Work out the finished part from the listing and answer in its coordinate system (mm). Face numbers are marked on the shaded views. A direction names the side the tool comes from. Coordinates: 2 decimals unless noted, no trailing zeros. Loops run counter-clockwise (first coordinate to the right, second up) from the corner with the lowest first, then second, coordinate; pieces in that order, holes last.
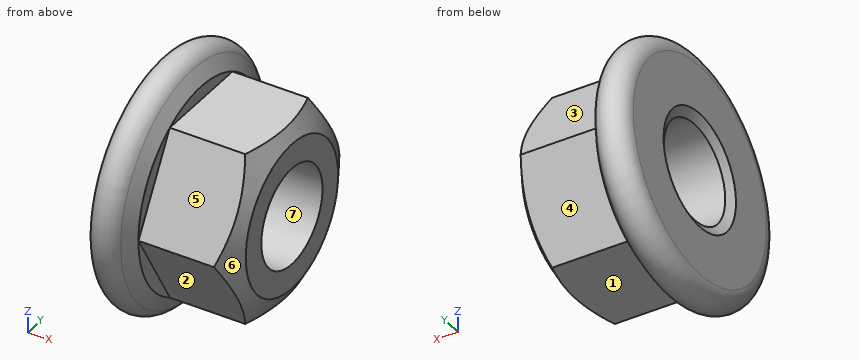
Autodesk Inventor part; units mm, degrees
ref_plane "Work Plane1" through (45.1755, 0, 0) normal (0, 0, -1) x (-1, 0, 0)
ref_plane "YZ Plane" through (0, 0, 0) normal (1, 0, 0) x (0, 1, 0)
ref_plane "XZ Plane" through (0, 0, 0) normal (0, 1, 0) x (-1, 0, 0)
sketch "Esquisse1" plane through (0, 0, 0) normal (0, 0, 1) x (1, 0, 0)
  line L0 (-3.6634, 0) -> (19.1606, 0)
  line L1 (4.9438, 12.1244) -> (3.9187, 13.9)
  line L2 (4.9438, 12.1244) -> (15.9, 12.1244) construction
  line L3 (15.9, 12.1244) -> (15.9, 0) construction
  arc A0 (3.9187, 13.9) -> (0, 12.85) centre (2.1, 12.85) ccw
  line L4 (4.9438, 12.1244) -> (4.9438, 0)
  line L5 (0, -3.0807) -> (0, 18.4841)
  point P0 (0, 0)
  dimension "d2" = 24.2487
  dimension "d4" = 29.9
  dimension "d5" = 2.1
  dimension "d15" = 15.9
  dimension "d16" = 30
revolve "Anneau" add sketch "Esquisse1" angle 360 about axis through (-10, 0, 0) along (1, 0, 0)
sketch "Esquisse2" plane through (0, 0, 0) normal (-1, 0, 0) x (0, 0, 1)
  circle A0 centre (0, 0) radius 4.9
  line L0 (-10.5, -6.0622) -> (-10.5, 6.0622)
  line L1 (-10.5, 6.0622) -> (0, 12.1244)
  line L2 (0, 12.1244) -> (10.5, 6.0622)
  line L3 (10.5, 6.0622) -> (10.5, -6.0622)
  line L4 (10.5, -6.0622) -> (0, -12.1244)
  line L5 (0, -12.1244) -> (-10.5, -6.0622)
  circle A1 centre (0, 0) radius 12.85
  dimension "d6" = 24.2487
extrude "Corps" add sketch "Esquisse2" against normal blind 15.9 contours A0 | L0 L1 L2 L3 L4 L5
sketch "Esquisse3" plane through (0, 0, 0) normal (0, 0, 1) x (1, 0, 0)
  line L0 (4.9438, 12.1244) -> (15.9, 12.1244)
  line L1 (15.9, 6.0622) -> (15.9, 12.1244)
  line L2 (0, -12.85) -> (0, 12.85)
  line L3 (-3.18, 0) -> (19.08, 0)
  line L4 (14.0529, 12.1244) -> (15.9, 8.925)
  dimension "d10" = 30
  dimension "d11" = 17.85
revolve "Chanfrein1" cut sketch "Esquisse3" angle 360 about axis through (-10, 0, 0) along (1, 0, 0)
sketch "Esquisse4" plane through (0, 0, 0) normal (-1, 0, 0) x (0, 0, 1)
  line L0 (-20.93, 0) -> (20.93, 0)
  line L1 (0, 20.93) -> (0, -20.93)
  point P0 (0, 0)
hole "Filetage" at (0, 0, 0) direction (1, 0, 0) diameter 11.835 end through all
chamfer "Chanfrein2" distance 1.0825 angle 30 1 edges at (0, 0, -5.9175) measured on face at (0, 10.4003, -1.2628)
ref_plane "Work Plane1" through (45.1755, 0, 0) normal (0, 0, -1) x (-1, 0, 0)
equation "\"d2\" = 1.1547 * SW"
equation "\"d4\" = LADI"
equation "\"d5\" = PHH"
equation "\"d15\" = KOH"
equation "\"d16\" = KEWI"
equation "\"d6\" = 1.1547 * SW"
equation "\"d7\" = KOH"
equation "\"d10\" = ANG1"
equation "\"d11\" = SW0"
equation "\"d12\" = -0.5 * GD1 + 0.5 * NND"
equation "\"d42\" = -0.5 * GD1 + 0.5 * NND"
equation "\"ANG1\" = 30deg"
equation "\"KEWI\" = 30deg"
equation "\"NND\" = 14"
equation "\"LADI\" = 29.9"
equation "\"SW\" = 21"
equation "\"PHH\" = 2.1"
equation "\"KOH\" = 15.9"
equation "\"SW0\" = 0.85 * SW"
equation "\"d1\" = LADI"
equation "\"d3\" = PHH"
equation "\"GUL\" = 0.541266 * PTC"
equation "\"THREADDIA\" = 14"
equation "\"TOA\" = 30deg"
equation "\"PTC\" = 2"
equation "\"GAL\" = 0.541266 * PTC"
equation "\"E0\" = 1.155 * SW"
properties part number "ANSI B18.16.3M - M14 x 2 Type de métal" material "Acier, doux"
1. A cutting plane is placed at C-C, the plane x = 1. Give the vertices of the cut face in (y, z) (1 decimal), then the cut area to 3 significant figures.
2. Straight lines are drawn through the part: probe 1 along Y at (x, z) = (10.5, 0); probe 2 along Z at (x, y) = (6.25, 0); probe 3 along X at (y, z) = (-9.5, -7). For each, find the intervals that lie inside material, in ascending order.
3. Determine the mould class of the marked faces 5, 6 and 7 for opening direction Z: released by +Z, released by -Z, zero draft, split by the parting line, or undercut.
4. A cutting plane is placed at A-A, the plane x = 9.75. Give the vertices of the cut face in (y, z) (1 decimal).
5. A cutting plane is placed at D-D, the plane x = 3.5. Give the vertices of the cut face in (y, z) (1 decimal), then the cut area to 3 significant figures.
6. Each of these flat-tipped pins is pushed along its axis until it touches: P1, Ø5, axis at y = 1, z = -1, coming from the -X side; P2, Ø8, axis at x = 9, y = -11.5, coming from the +Z side; P3, Ø5, axis at x = 12.5, z = 9, coming from the +Y side; P4, Ø1.5, axis at y = 10.5, z = 3.5, coming from the +X side. Where does it stop, or does it pass through?
7. For the marked faces 1, 2, 3 and 4, determine the directions among +Z, -Z, +X, -X, +Y, -Y from which every point of the face is accessible in a straight line to the end or side of a thin tool.
Answers below:
1. outline: circle Ø29.3 at (0, 0); hole circle Ø11.8 at (0, 0)
1. area: 563 mm2
2. probe 1: y = -12.12 to -5.92, 5.92 to 12.12
2. probe 2: z = -10.5 to -5.92, 5.92 to 10.5
2. probe 3: x = 0 to 4.94
3. face 5: released by +Z
3. face 6: split by the parting line
3. face 7: undercut
4. outline: (-12.1, 0) - (-6.1, -10.5) - (6.1, -10.5) - (12.1, 0) - (6.1, 10.5) - (-6.1, 10.5) - close; hole circle Ø11.8 at (0, 0)
5. outline: circle Ø28.8 at (0, 0); hole circle Ø11.8 at (0, 0)
5. area: 543 mm2
6. P1: passes through
6. P2: stops at z = 8.01
6. P3: stops at y = 8.37
6. P4: stops at x = 15.1
7. face 1: -Z, +X, +Y, -Y
7. face 2: -Z, +X, -Y
7. face 3: +Z, +X, +Y
7. face 4: -Z, +X, +Y
